```python
from build123d import *

# Parameters (mm, degrees)
SKETCH1_R           = 2.5
SKETCH1_R_2         = 2
BOSS_EXTRUDE1_DEPTH = 2.2


with BuildPart() as part:
    # Sketch1 → Boss-Extrude1 (new body)
    with BuildSketch(Plane(origin=(0, 0, 0), x_dir=(1, 0, 0), z_dir=(0, 1, 0))):
        with BuildLine():
            Line((-47.65, -142.074373129), (-47.65, -106.264514288))
            ThreePointArc((-47.65, -106.264514288), (-46.185533906, -102.728980382), (-42.65, -101.264514288))
            Line((-42.65, -101.264514288), (42.65, -101.264514288))
            ThreePointArc((42.65, -101.264514288), (46.185533906, -102.728980382), (47.65, -106.264514288))
            Line((47.65, -106.264514288), (47.65, -142.074373129))
            ThreePointArc((47.65, -142.074373129), (48.492330213, -143.705262661), (50.309800664, -143.962404666))
            ThreePointArc((50.309800664, -143.962404666), (132.068874077, -76.25), (149.829999963, 28.411636898))
            ThreePointArc((149.829999963, 28.411636898), (148.698573228, 29.857041477), (146.865016356, 29.771076074))
            Line((146.865016356, 29.771076074), (115.852768895, 11.866146654))
            ThreePointArc((115.852768895, 11.866146654), (112.058673669, 11.366644541), (109.022641876, 13.696273673))
            Line((109.022641876, 13.696273673), (66.372641876, 87.568240616))
            ThreePointArc((66.372641876, 87.568240616), (65.873139763, 91.362335841), (68.202768895, 94.398367635))
            Line((68.202768895, 94.398367635), (99.215016356, 112.303297055))
            ThreePointArc((99.215016356, 112.303297055), (100.206243015, 113.848221184), (99.520199298, 115.550767768))
            ThreePointArc((99.520199298, 115.550767768), (0, 152.5), (-99.520199298, 115.550767768))
            ThreePointArc((-99.520199298, 115.550767768), (-100.206243015, 113.848221184), (-99.215016356, 112.303297055))
            Line((-99.215016356, 112.303297055), (-68.202768895, 94.398367635))
            ThreePointArc((-68.202768895, 94.398367635), (-65.873139763, 91.362335841), (-66.372641876, 87.568240616))
            Line((-66.372641876, 87.568240616), (-109.022641876, 13.696273673))
            ThreePointArc((-109.022641876, 13.696273673), (-112.058673669, 11.366644541), (-115.852768895, 11.866146654))
            Line((-115.852768895, 11.866146654), (-146.865016356, 29.771076074))
            ThreePointArc((-146.865016356, 29.771076074), (-148.698573228, 29.857041477), (-149.829999963, 28.411636898))
            ThreePointArc((-149.829999963, 28.411636898), (-132.068874077, -76.25), (-50.309800664, -143.962404666))
            ThreePointArc((-50.309800664, -143.962404666), (-48.492330213, -143.705262661), (-47.65, -142.074373129))
        make_face()
        with Locations((-15, -85.914514288)):
            Circle(SKETCH1_R, mode=Mode.SUBTRACT)
        with Locations((15, -85.914514288)):
            Circle(SKETCH1_R, mode=Mode.SUBTRACT)
        with Locations((105.474308644, -89.763133948)):
            Circle(SKETCH1_R_2, mode=Mode.SUBTRACT)
        with Locations((130.474308644, -46.461863758)):
            Circle(SKETCH1_R_2, mode=Mode.SUBTRACT)
        with Locations((93.782965693, -83.013133948)):
            Circle(SKETCH1_R_2, mode=Mode.SUBTRACT)
        with Locations((118.782965693, -39.711863758)):
            Circle(SKETCH1_R_2, mode=Mode.SUBTRACT)
        with Locations((99.159908733, -57.25)):
            Circle(SKETCH1_R_2, mode=Mode.SUBTRACT)
        with Locations((39.404155872, -22.75)):
            Circle(SKETCH1_R_2, mode=Mode.SUBTRACT)
        with Locations((-99.159908733, -57.25)):
            Circle(SKETCH1_R_2, mode=Mode.SUBTRACT)
        with Locations((-93.782965693, -83.013133948)):
            Circle(SKETCH1_R_2, mode=Mode.SUBTRACT)
        with Locations((-105.474308644, -89.763133948)):
            Circle(SKETCH1_R_2, mode=Mode.SUBTRACT)
        with Locations((-130.474308644, -46.461863758)):
            Circle(SKETCH1_R_2, mode=Mode.SUBTRACT)
        with Locations((-118.782965693, -39.711863758)):
            Circle(SKETCH1_R_2, mode=Mode.SUBTRACT)
        with Locations((-39.404155872, -22.75)):
            Circle(SKETCH1_R_2, mode=Mode.SUBTRACT)
        with Locations((0, 114.5)):
            Circle(SKETCH1_R_2, mode=Mode.SUBTRACT)
        with Locations((-25, 122.724997706)):
            Circle(SKETCH1_R_2, mode=Mode.SUBTRACT)
        with Locations((-25, 136.224997706)):
            Circle(SKETCH1_R_2, mode=Mode.SUBTRACT)
        with Locations((25, 136.224997706)):
            Circle(SKETCH1_R_2, mode=Mode.SUBTRACT)
        with Locations((25, 122.724997706)):
            Circle(SKETCH1_R_2, mode=Mode.SUBTRACT)
        with Locations((0, 45.5)):
            Circle(SKETCH1_R_2, mode=Mode.SUBTRACT)
        with Locations((15, -56.414514288)):
            Circle(SKETCH1_R, mode=Mode.SUBTRACT)
        with Locations((-15, -56.414514288)):
            Circle(SKETCH1_R, mode=Mode.SUBTRACT)
        with Locations((-56.356402516, 15.216876087)):
            Circle(SKETCH1_R, mode=Mode.SUBTRACT)
        with Locations((-81.904151928, 29.966876087)):
            Circle(SKETCH1_R, mode=Mode.SUBTRACT)
        with Locations((-66.904151928, 55.947638201)):
            Circle(SKETCH1_R, mode=Mode.SUBTRACT)
        with Locations((-41.356402516, 41.197638201)):
            Circle(SKETCH1_R, mode=Mode.SUBTRACT)
        with Locations((41.356402516, 41.197638201)):
            Circle(SKETCH1_R, mode=Mode.SUBTRACT)
        with Locations((66.904151928, 55.947638201)):
            Circle(SKETCH1_R, mode=Mode.SUBTRACT)
        with Locations((81.904151928, 29.966876087)):
            Circle(SKETCH1_R, mode=Mode.SUBTRACT)
        with Locations((56.356402516, 15.216876087)):
            Circle(SKETCH1_R, mode=Mode.SUBTRACT)
    extrude(amount=BOSS_EXTRUDE1_DEPTH)


solid = part.part
```
Input: part model. Units: mm. Frame: model coordinates. A direction names the side the tool comes from. Give positions to 0.01 mm unless a question says otherwise; leave off trailing zeros. Write each loop counter-clockwise with the first axis right and the second up, starting at its lowest first coordinate (ties: lowest second). Pieces come first, ordered by that corner, then holes. Notation, with made-up numbers: (-26.75, -7) - (15.25, -7) arc R16 cw to (15.25, 6) - close; hole circle Ø10 at (38, -19.75). An arc over 180 degrees is marked (long way). Write item = value, one per line. Start each with the question number.
1) Pin query (flat end, axial travel): pin 1 (0.7 mm diameter, centred on y = 1, z = 122.5, fed in from -X); pin 2 (0.7 mm diameter, centred on y = 1, z = 116, fed in from +X); pin 3 (1 mm diameter, centred on y = 1.5, z = -107, fed in from +X). Return the tip coordinate at first contact, or that it passes through.
2) Reachability of faces 5 (the face through (87.996, 1.085, -50.115)), 6 (the face through (83.492, 1.085, -103.225)), 7 (the face through (-2, 2.2, -6)), 8 (the face through (-131.14, 1.08, -20.69)) from +Z, -Z, +X, -X, +Y, -Y: full face, straight path, thin tool, end or side. Return the list, or none.
3) Draft query along Z for faces 1 (the face through (-2, 0, -6)), 2 (the face through (131.303, 1.085, 77.561)), 3 (the face through (-83.93, 1.08, -103.48)), 4 (the face through (1.518, 1.085, -152.492)). Return one class per face: pulls with the +Z half, pulls with the -Z half, needs draft (parallel to the pull), parting line crosses it, or undercut.
4) Cut plane B-B (y = 1.5). Give the number of separate pieces and of enclosed holes in the cut face, and give its area (3 significant figures).
5) Cut plane A-A (x = 124.5). Return loops of the section in (y, z), and give its area (3 significant figures).
6) Material intervals for L1, parallel to Z at x = -0.5, y = 1.9; L2, parallel to Z at x = 15, y = 0.8; L3, parallel to X at y = 1.55, z = 57.25, sorted ascending. Write a range as [from, to].
Answers follow:
q1.pin_1 = -91.3
q1.pin_2 = 99.4
q1.pin_3 = 90.9
q2.face_5 = +Y, -Y
q2.face_6 = +X, +Y, -Y
q2.face_7 = +Z, -Z, +X, -X, +Y
q2.face_8 = -Z, +Y, -Y
q3.face_1 = needs draft
q3.face_2 = parting line crosses it
q3.face_3 = undercut
q3.face_4 = pulls with the -Z half
q4.separate_pieces = 1
q4.enclosed_holes = 30
q4.area = 58,700 mm^2
q5.outline = (0, -16.86) - (2.2, -16.86) - (2.2, 88.07) - (0, 88.07) - close
q5.area = 231 mm^2
q6.L1 = [-152.5, -116.44], [-112.56, -47.44], [-43.56, 101.26]
q6.L2 = [-151.76, 53.91], [58.91, 83.41], [88.41, 101.26]
q6.L3 = [-141.35, -101.16], [-97.16, -17.36], [-12.64, 12.64], [17.36, 97.16], [101.16, 141.35]
